Verification items for the finished model (mm, model axes). A direction names the side the tool comes from. Round coordinates to 2 decimals unless told otherwise and drop trailing zeros. Write each loop counter-clockwise with the first axis right and the second up, starting at its lowest first coordinate (ties: lowest second). Pieces come first, ordered by that corner, then holes. Notation, with made-up numbers: M -9.75,-26.5 L 47.25,-26.5 A29 ccw 47.25,-6.5 Z; hole C -34.75,84 d4. An arc over 180 degrees is marked long. Use a Markdown table: item, result. Add a question column.
from build123d import *

# Parameters (mm, degrees)
SKETCH1_R           = 88.9
BOSS_EXTRUDE1_DEPTH = 50.8
SKETCH2_R           = 82.55
CUT_EXTRUDE1_DEPTH  = 44.45
SKETCH3_R           = 45.72
SKETCH3_R_2         = 1.397
CUT_EXTRUDE2_DEPTH  = 7.35


with BuildPart() as part:
    # Sketch1 → Boss-Extrude1 (new body)
    with BuildSketch(Plane(origin=(0, 0, 0), x_dir=(1, 0, 0), z_dir=(0, 1, 0))):
        Circle(SKETCH1_R)
    extrude(amount=BOSS_EXTRUDE1_DEPTH)

    # Sketch2 → Cut-Extrude1 (cut)
    with BuildSketch(Plane(origin=(0, 50.8, 0), x_dir=(1, 0, 0), z_dir=(0, 1, 0))):
        Circle(SKETCH2_R)
    extrude(amount=-CUT_EXTRUDE1_DEPTH, mode=Mode.SUBTRACT)

    # Sketch3 → Cut-Extrude2 (cut, through all)
    with BuildSketch(Plane(origin=(0, 6.35, 0), x_dir=(1, 0, 0), z_dir=(0, 1, 0))):
        Circle(SKETCH3_R)
        with Locations((0, 52.07)):
            Circle(SKETCH3_R_2)
        with Locations((26.035, 45.093942775)):
            Circle(SKETCH3_R_2)
        with Locations((45.093942775, 26.035)):
            Circle(SKETCH3_R_2)
        with Locations((52.07, 0)):
            Circle(SKETCH3_R_2)
        with Locations((45.093942775, -26.035)):
            Circle(SKETCH3_R_2)
        with Locations((26.035, -45.093942775)):
            Circle(SKETCH3_R_2)
        with Locations((0, -52.07)):
            Circle(SKETCH3_R_2)
        with Locations((-26.035, -45.093942775)):
            Circle(SKETCH3_R_2)
        with Locations((-45.093942775, -26.035)):
            Circle(SKETCH3_R_2)
        with Locations((-52.07, 0)):
            Circle(SKETCH3_R_2)
        with Locations((-45.093942775, 26.035)):
            Circle(SKETCH3_R_2)
        with Locations((-26.035, 45.093942775)):
            Circle(SKETCH3_R_2)
    extrude(amount=-CUT_EXTRUDE2_DEPTH, mode=Mode.SUBTRACT)


solid = part.part
1. Cross-section at B-B on x = -66. Enter the section's corners in (y, z).
2. Cross-section at A-A on z = -20.5. Enter the section's corners in (x, y), plus the area to 3 significant figures.
3. Access from +Z, -Z, +X, -X, +Y, -Y to the whole of each face (thin tool, end or side, straight path). Record for faces 4 (the cylindrical face through (43.61, 3.22, -13.73)), 5 (the cylindrical face through (-17.895, 28.886, 80.587)).
4. Scan lines: line 1 along X through (y, z) = (3, 0); line 2 along X through (y, z) = (37.5, 0). Record each from-to range of solid material in increasing order. Write a range as from..to.
5. Depth check by flat-ended pin: pin 1 Ø3.5 at (x, z) = (45.09, -26.04) entering from +Y; pin 2 Ø4 at (x, y) = (20, 41) entering from -Z; pin 3 Ø3 at (y, z) = (30.5, 11) entering from +X; pin 4 Ø1.7 at (x, z) = (-45.09, 26.04) entering from +Y. Enter the tip coordinate at first touch or a pass-through.
6. Cross-section at D-D on x = -9.5. Enter the section's corners in (y, z), plus the area to 3 significant figures.
7. Release check for a two-part mould opening along Z. For faces 1 (the cylindrical face through (84.795, 25.044, -26.703)), 2 (the flat face through (36, 6.35, 36)), 3 (the flat face through (-41, 0, -21)) record: +Z half, -Z half, draft (parallel to the pull), parting line (faces both ways), or undercut.
8. Cross-section at C-C on y = 23. Enter the section's corners in (x, z), plus the area to 3 significant figures.
Answer:
| question | item | result |
|---|---|---|
| 1 | outline | M 0,-59.56 L 50.8,-59.56 L 50.8,-49.58 L 6.35,-49.58 L 6.35,49.58 L 50.8,49.58 L 50.8,59.56 L 0,59.56 Z |
| 2 | outline | M -86.5,0 L -40.87,0 L -40.87,6.35 L -79.96,6.35 L -79.96,50.8 L -86.5,50.8 Z; M 40.87,0 L 86.5,0 L 86.5,50.8 L 79.96,50.8 L 79.96,6.35 L 40.87,6.35 Z |
| 2 | area | 1,160 mm^2 |
| 3 | face 4 | +Y, -Y |
| 3 | face 5 | +Y |
| 4 | line 1 | x = -88.9..-53.47, -50.67..-45.72, 45.72..50.67, 53.47..88.9 |
| 4 | line 2 | x = -88.9..-82.55, 82.55..88.9 |
| 5 | pin 1 | stops at y = 6.35 |
| 5 | pin 2 | stops at z = -87.06 |
| 5 | pin 3 | stops at x = 88.39 |
| 5 | pin 4 | passes through |
| 6 | outline | M 0,-88.39 L 50.8,-88.39 L 50.8,-82 L 6.35,-82 L 6.35,-44.72 L 0,-44.72 Z; M 0,44.72 L 6.35,44.72 L 6.35,82 L 50.8,82 L 50.8,88.39 L 0,88.39 Z |
| 6 | area | 1,120 mm^2 |
| 7 | face 1 | parting line |
| 7 | face 2 | undercut |
| 7 | face 3 | draft |
| 8 | outline | C 0,0 d177.8; hole C 0,0 d165.1 |
| 8 | area | 3,420 mm^2 |
